```python
from build123d import *

# Parameters (mm, degrees)
F0_W           = 32
F0_H           = 32
F1_DEPTH       = 7
F3_D           = 7
F3_CSINK_D     = 10
F3_CSINK_ANGLE = 60


with BuildPart() as f1:
    # F0 (on Top) → F1 (new body)
    with BuildSketch(Plane.XY):
        Rectangle(F0_W, F0_H)
    extrude(amount=F1_DEPTH)

    # F3 (through all)
    with Locations(Plane.XY.offset(7)):
        with Locations((-8, 0), (8, 0)):
            CounterSinkHole(F3_D / 2, F3_CSINK_D / 2, counter_sink_angle=F3_CSINK_ANGLE)


solid = f1.part
```
The listing builds one solid part. Answer for the finished solid, in the listing's coordinates (mm). Round coordinates to 2 decimals unless told otherwise and drop trailing zeros. Loops run counter-clockwise (first coordinate to the right, second up) from the corner with the lowest first, then second, coordinate; pieces in that order, holes last. Notation, with made-up numbers: (20, -12) -> (65, -12) arc R34 cw to (65, 24) -> close; hole circle Ø9 at (34, 64). An arc over 180 degrees is marked (long way). Use one line per item in the form item = value.
1. The part is cut by section A-A on x = -8. Determine the outline of the cut face in (y, z).
Answer key:
outline = (-16, 0) -> (-3.5, 0) -> (-3.5, 4.4) -> (-5, 7) -> (-16, 7) -> close; (3.5, 0) -> (16, 0) -> (16, 7) -> (5, 7) -> (3.5, 4.4) -> close
2. For a pull along Y with two mould halves and no side action, classify faces 1 (the flat face through (0, 16, 3)), 2 (the cylindrical face through (-4.503, 0.154, 2.17)), 3 (the cylindrical face through (11.497, 0.154, 2.17)), 4 (the flat face through (-16, 0, 3)) as released by +Y, released by -Y, zero draft, split by the parting line, or undercut.
Answer key:
face_1 = released by +Y
face_2 = undercut
face_3 = undercut
face_4 = zero draft
3. The part is cut by section C-C on z = 1.5. Determine the outline of the cut face in (x, y), and give its area (3 significant figures).
Answer key:
outline = (-16, -16) -> (16, -16) -> (16, 16) -> (-16, 16) -> close; hole circle Ø7 at (-8, 0); hole circle Ø7 at (8, 0)
area = 947 mm²
4. The part is cut by section D-D on z = 5.75. Determine the outline of the cut face in (x, y), and give its area (3 significant figures).
Answer key:
outline = (-16, -16) -> (16, -16) -> (16, 16) -> (-16, 16) -> close; hole circle Ø8.56 at (-8, 0); hole circle Ø8.56 at (8, 0)
area = 909 mm²
5. A flat-ended cylindrical pin translates along its axis: pin 1 Ø11 at (x, y) = (-8, 0) entering from -Z. Find the tip coordinate at first contact, or state that the pin passes through.
Answer key:
pin_1 = 0
6. The part is cut by section B-B on y = 0. Determine the outline of the cut face in (x, z).
Answer key:
outline = (-16, 0) -> (-11.5, 0) -> (-11.5, 4.4) -> (-13, 7) -> (-16, 7) -> close; (-4.5, 0) -> (4.5, 0) -> (4.5, 4.4) -> (3, 7) -> (-3, 7) -> (-4.5, 4.4) -> close; (11.5, 0) -> (16, 0) -> (16, 7) -> (13, 7) -> (11.5, 4.4) -> close
7. Find the intervals of material crossed by probe 1 along X at (y, z) = (0, 3.05); probe 2 along Y at (x, z) = (-8, 1.5); probe 3 along X at (y, z) = (-3.5, 5.25) (3 decimals), in increasing order. Write a range as [from, to].
Answer key:
probe_1 = [-16, -11.5], [-4.5, 4.5], [11.5, 16]
probe_2 = [-16, -3.5], [3.5, 16]
probe_3 = [-16, -9.915], [-6.085, 6.085], [9.915, 16]
